The drawing under review shows one solid part. Ordinate dimensions are in mm from its lowest x, y, z. Coordinates: 2 decimals unless noted, no trailing zeros. Loops run counter-clockwise (first coordinate to the right, second up) from the corner with the lowest first, then second, coordinate; pieces in that order, holes last. Notation, with made-up numbers: M 3.5,21.5 L 61.5,21.5 A13 ccw 61.5,36.5 Z; hole C 82.5,36.5 d10. An arc over 180 degrees is marked long. Put each result on its own line as item: value.
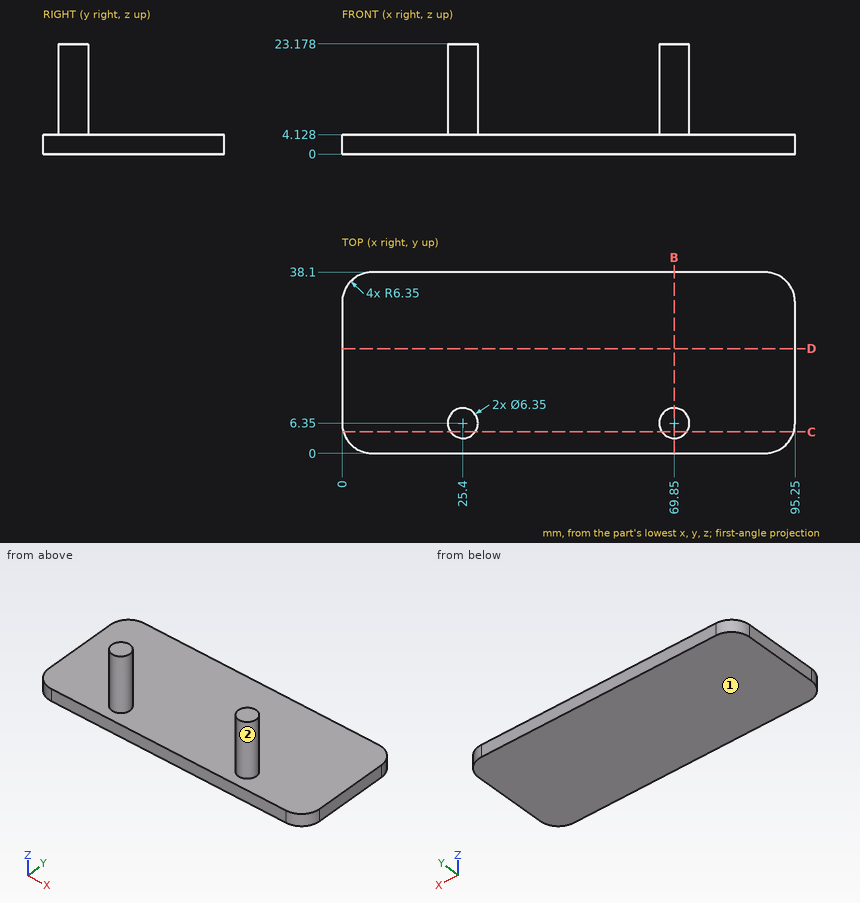
(1) Add section D-D (y = 22). Write out the cut boundary in (x, z).
Determined:
outline: M 0,0 L 95.25,0 L 95.25,4.13 L 0,4.13 Z
(2) For pin 1 (12 mm diameter, centred on x = 47, y = 8.5, fed in from +Z); pin 2 (4 mm diameter, centred on x = 24, z = 19.5, fed in from +Y) (1 decimal); pin 3 (1.5 mm diameter, centred on x = 67, z = 19.5, fed in from +Y); pin 4 (6 mm diameter, centred on y = 9.5, z = 4.5, fed in from +X), all flat-tipped, find the tip position at first contact; note any pin that passes through.
Determined:
pin 1: stops at z = 4.13
pin 2: stops at y = 9.5
pin 3: stops at y = 8.73
pin 4: stops at x = 95.25
(3) Draft analysis for pull direction X (two halves, no side actions). For the marked faces 1 and 2, state which applies: +X half, -X half, draft (parallel to the pull), parting line (faces both ways), or undercut.
Determined:
face 1: draft
face 2: undercut
(4) Wall thickness on line 1 along Z through (x, y) = (12, 16); line 2 along Y through (x, z) = (68, 18.75): over which ranges is each line inside the solid? List them lowest first. Write a range as [from, to].
Determined:
line 1: z = [0, 4.13]
line 2: y = [3.77, 8.93]
(5) Add section C-C (y = 4.5). Write out the cut boundary in (x, z) (1 decimal).
Determined:
outline: M 0.3,0 L 95,0 L 95,4.1 L 72.4,4.1 L 72.4,23.2 L 67.3,23.2 L 67.3,4.1 L 28,4.1 L 28,23.2 L 22.8,23.2 L 22.8,4.1 L 0.3,4.1 Z
(6) Add section B-B (x = 69.85). Write out the cut boundary in (y, z) (1 decimal), plus the area to 3 significant figures.
Determined:
outline: M 0,0 L 38.1,0 L 38.1,4.1 L 9.5,4.1 L 9.5,23.2 L 3.2,23.2 L 3.2,4.1 L 0,4.1 Z
area: 278 mm^2
